Check sheet for the drawn part. Datum: minimum x, y, z corner. Units: mm. Coordinates: 2 decimals unless noted, no trailing zeros. Order: outer loops, then holes, each group sorted by start corner. A loop starts at its lowest first (then second) coordinate and runs counter-clockwise, first axis right, second up.
Q1. Cross-section at A-A, the plane y = 201. Record the boundary of the cut face in (x, z).
Q2. Thickness scan on line 1 (X direction, y = 141, z = 1.5); line 2 (X direction, y = 165.5, z = 2); line 3 (Y direction, x = 65, z = 3.25). Record the ranges inside material, lowest first.
Q3. Depth check by flat-ended pin: P1, Ø10, axis at x = 47, y = 98, coming from the -Z side; P2, Ø11.5, axis at x = 120.65, y = 66.675, coming from the -Z side. Enter the tip coordinate at first touch or a pass-through.
Q4. Cross-section at D-D, the plane x = 159.5. Record the boundary of the cut face in (y, z).
Q5. Cross-section at B-B, the plane x = 120.65. Count the separate pieces of the cut face and the enclosed holes in it, and give its area (3 significant figures).
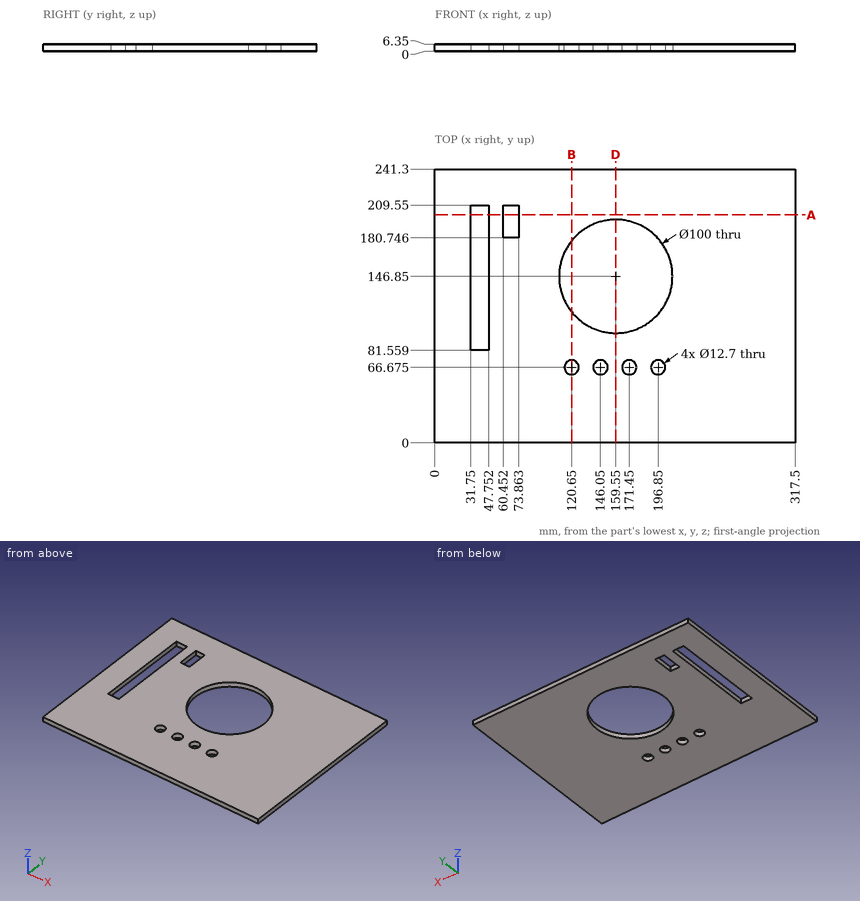
Check values:
1. outline: (0, 0) - (31.75, 0) - (31.75, 6.35) - (0, 6.35) - close; (47.75, 0) - (60.45, 0) - (60.45, 6.35) - (47.75, 6.35) - close; (73.86, 0) - (317.5, 0) - (317.5, 6.35) - (73.86, 6.35) - close
2. line 1: x = 0 to 31.75, 47.75 to 109.89, 209.21 to 317.5
2. line 2: x = 0 to 31.75, 47.75 to 113.16, 205.94 to 317.5
2. line 3: y = 0 to 180.75, 209.55 to 241.3
3. P1: stops at z = 0
3. P2: passes through
4. outline: (0, 0) - (96.85, 0) - (96.85, 6.35) - (0, 6.35) - close; (196.85, 0) - (241.3, 0) - (241.3, 6.35) - (196.85, 6.35) - close
5. separate pieces: 3
5. enclosed holes: 0
5. area: 1,050 mm2
